Part model, mm, in its own coordinate system. A direction names the side the tool comes from. Give positions to 0.01 mm unless a question says otherwise; leave off trailing zeros. Write each loop counter-clockwise with the first axis right and the second up, starting at its lowest first coordinate (ties: lowest second). Pieces come first, ordered by that corner, then holes. Notation, with made-up numbers: M -38,3.25 L -7,3.25 A8 ccw -7,14.25 Z; hole C -35,22.5 d5. An arc over 180 degrees is marked long. Use CSV: the item, a comma, the result in double quotes. Start each with the question number.
Item 1: Pin check, flat tips, straight feed: pin 1 (2 mm diameter, centred on y = 0, z = -52, fed in from -X); pin 2 (12 mm diameter, centred on x = -64.5, z = -14, fed in from -Y); pin 3 (12 mm diameter, centred on x = -66.5, z = -5, fed in from -Y); pin 4 (4.5 mm diameter, centred on y = 31.82, z = 31.82, fed in from +X). Stop position of each tip, or through.
Item 2: Drill centre lines: line 1 (Y direction, x = 12.7, z = 0); line 2 (Z direction, x = -80, y = -35.5) (3 decimals); line 3 (Y direction, x = -21, z = -17.5). Where is each one in solid material? Low to high. Write a range as [from, to].
Item 3: Which spindle directions (+Z, -Z, +X, -X, +Y, -Y) get a long thin tool onto all of the face, cutting with end or side? Do faces 4 (the cylindrical face through (11.73, 31.24, -6.94)), 5 (the cylindrical face through (-57.2, -14.718, 46.737)). Say none if no direction does.
Item 4: Cut at D-D (z = 43.5). List the corners of the cut face in (x, y).
Item 5: Cut at C-C (x = -7). List the corners of the cut face in (y, z), then the cut area to 3 significant figures.
Item 6: Cut at A-A (z = -24.5). List the corners of the cut face in (x, y), then the cut area to 3 significant figures.
Item 7: Mould opens along Y. For faces 1 (the cylindrical face through (11.67, -32.82, -30.51)), 2 (the cylindrical face through (-57.128, 48.794, 25.379)), 3 (the flat face through (-126, -37, -33)) say: released by +Y, released by -Y, zero draft, split by the parting line, or undercut.
Item 8: Cut at B-B (y = 22). List the corners of the cut face in (x, z), then the cut area to 3 significant figures.
from build123d import *

# Parameters (mm, degrees)
AXIAL_START        = 9.7
SKETCH2_R          = 1.65
AXIAL_HOLES_DEPTH  = 4
CUT_EXTRUDE2_START = -126
SKETCH3_R          = 1.25
CUT_EXTRUDE2_DEPTH = 6


with BuildPart() as part:
    # Axial profile (mm) → Full revolution (revolve)
    with BuildSketch(Plane.XY, mode=Mode.PRIVATE) as full_revolution_sk:
        Polygon((-126, 49), (9.7, 49), (9.7, 32), (13.7, 32), (13.7, 55), (-126, 55), align=None)
    revolve(full_revolution_sk.sketch.rotate(Axis((-110, 0, 0), (1, 0, 0)), 90), axis=Axis((-110, 0, 0), (1, 0, 0)))

    # Sketch2 → Axial holes (cut)
    with BuildSketch(Plane(origin=(0, 0, 0), x_dir=(0, 0, -1), z_dir=(1, 0, 0)).offset(AXIAL_START)):
        with Locations((-31.819805153, 31.819805153)):
            Circle(SKETCH2_R)
        with Locations((-31.819805153, -31.819805153)):
            Circle(SKETCH2_R)
        with Locations((31.819805153, -31.819805153)):
            Circle(SKETCH2_R)
        with Locations((31.819805153, 31.819805153)):
            Circle(SKETCH2_R)
    extrude(amount=AXIAL_HOLES_DEPTH, mode=Mode.SUBTRACT)

    # Sketch3 → Cut-Extrude2 (cut)
    with BuildSketch(Plane(origin=(0, 0, 0), x_dir=(0, 0, -1), z_dir=(1, 0, 0)).offset(CUT_EXTRUDE2_START)):
        with Locations((0, 52)):
            Circle(SKETCH3_R)
        with Locations((-52, 0)):
            Circle(SKETCH3_R)
        with Locations((0, -52)):
            Circle(SKETCH3_R)
        with Locations((52, 0)):
            Circle(SKETCH3_R)
    extrude(amount=CUT_EXTRUDE2_DEPTH, mode=Mode.SUBTRACT)


solid = part.part
Worked answers:
1,pin 1,"stops at x = -120"
1,pin 2,"stops at y = -54.42"
1,pin 3,"stops at y = -55"
1,pin 4,"stops at x = 13.7"
2,line 1,"y = [-55, -32], [32, 55]"
2,line 2,"z = [-42.009, -33.775], [33.775, 42.009]"
2,line 3,"y = [-52.14, -45.77], [45.77, 52.14]"
3,face 4,"+X, -X"
3,face 5,"-X"
4,outline,"M -126,-33.66 L 13.7,-33.66 L 13.7,33.66 L -126,33.66 L -126,22.56 L 9.7,22.56 L 9.7,-22.56 L -126,-22.56 Z"
5,outline,"C 0,0 d110; hole C 0,0 d98"
5,area,"1,960 mm^2"
6,outline,"M -126,-49.24 L 13.7,-49.24 L 13.7,-20.59 L 9.7,-20.59 L 9.7,-42.44 L -126,-42.44 Z; M -126,42.44 L 9.7,42.44 L 9.7,20.59 L 13.7,20.59 L 13.7,49.24 L -126,49.24 Z"
6,area,"2,080 mm^2"
7,face 1,"undercut"
7,face 2,"split by the parting line"
7,face 3,"zero draft"
8,outline,"M -126,-50.41 L 13.7,-50.41 L 13.7,-23.24 L 9.7,-23.24 L 9.7,-43.78 L -126,-43.78 Z; M -126,43.78 L 9.7,43.78 L 9.7,23.24 L 13.7,23.24 L 13.7,50.41 L -126,50.41 Z"
8,area,"2,020 mm^2"
